Study the drawing (mm; zero at the part's minimum x, y, z) and answer. A direction names the side the tool comes from. Round coordinates to 2 decimals unless told otherwise and drop trailing zeros. Order: outer loops, then holes, each group sorted by start corner. A loop starts at its lowest first (then second) coordinate and runs counter-clockwise, first axis right, second up. Notation, with made-up numbers: (64.5, 73.5) -> (100.5, 73.5) arc R23 cw to (100.5, 104.5) -> close; hole circle Ø7 at (-8, 46). An arc over 180 degrees is marked (long way). Use one line per item in the form item = value.
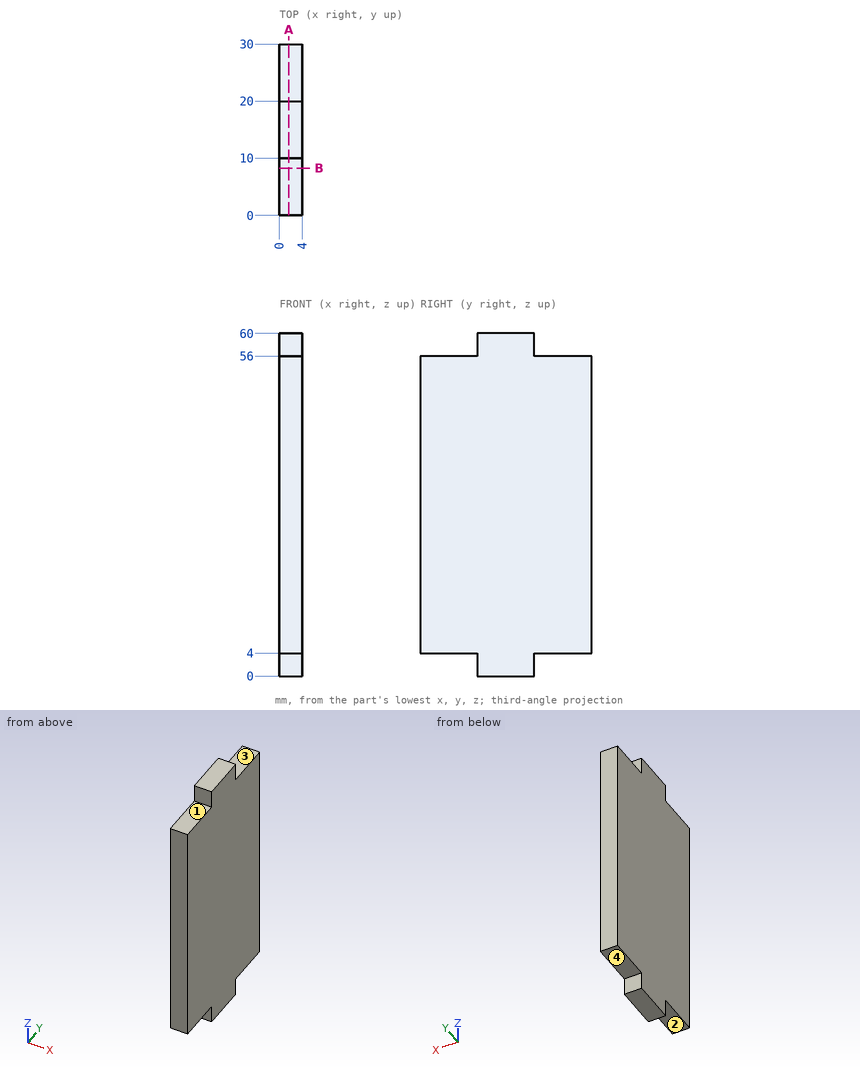
Item 1: For the marked faces 1, 2, 3 and 4, determine the directions among +Z, -Z, +X, -X, +Y, -Y from which every point of the face is accessible in a straight line to the end or side of a thin tool.
Findings:
face_1 = +Z, +X, -X, -Y
face_2 = -Z, +X, -X, -Y
face_3 = +Z, +X, -X, +Y
face_4 = -Z, +X, -X, +Y
Item 2: The part is cut by section A-A, the plane x = 1.65. Give the vertices of the cut face in (y, z).
Findings:
outline = (0, 4) -> (10, 4) -> (10, 0) -> (20, 0) -> (20, 4) -> (30, 4) -> (30, 56) -> (20, 56) -> (20, 60) -> (10, 60) -> (10, 56) -> (0, 56) -> close
Item 3: Consider line 1 along Z through (x, y) = (2.6, 24.25). Determine where the line is inside the solid, lowest interval first.
Findings:
line_1 = 4 to 56
Item 4: Flat-ended cylindrical pins translate along their axes: P1, Ø1.2, axis at x = 2, y = 24.5, coming from the -Z side; P2, Ø2, axis at x = 2.5, z = 2.5, coming from the +Y side; P3, Ø1.2, axis at x = 1.5, y = 3.5, coming from the +Z side. Find the tip coordinate at first contact, or state that the pin passes through.
Findings:
P1 = 4
P2 = 20
P3 = 56
Item 5: The part is cut by section B-B, the plane y = 8.25. Give the vertices of the cut face in (x, z).
Findings:
outline = (0, 4) -> (4, 4) -> (4, 56) -> (0, 56) -> close
